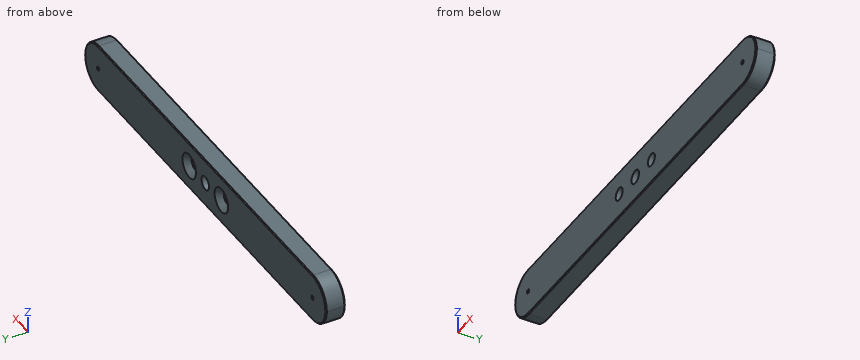
Autodesk Inventor part; units mm, degrees
ref_plane "YZ Plane" through (0, 0, 0) normal (1, 0, 0) x (0, 1, 0)
ref_plane "XZ Plane" through (0, 0, 0) normal (0, 1, 0) x (-1, 0, 0)
ref_plane "XY Plane" through (0, 0, 0) normal (0, 0, 1) x (1, 0, 0)
sketch "Sketch1" plane through (0, 0, 0) normal (0, 1, 0) x (-1, 0, 0)
  line L0 (-112.5, 12.5) -> (112.5, 12.5)
  line L1 (112.5, 12.5) -> (112.5, -12.5)
  line L2 (112.5, -12.5) -> (-112.5, -12.5)
  line L3 (-112.5, -12.5) -> (-112.5, 12.5)
  line L4 (-112.5, 12.5) -> (112.5, -12.5) construction
  line L5 (112.5, 12.5) -> (-112.5, -12.5) construction
  point P0 (0, 0)
  dimension "Length" = 225
  dimension "Width" = 25
extrude "Extrusion1" add sketch "Sketch1" along normal mid plane 10
sketch "Sketch2" plane through (0, 5, 0) normal (0, 1, 0) x (1, 0, 0)
  circle A0 centre (0, 0) radius 3.5
  dimension "d4" = 7
extrude "Extrusion2" cut sketch "Sketch2" against normal up to surface (10 mm away)
sketch "Sketch3" plane through (0, 5, 0) normal (0, 1, 0) x (1, 0, 0)
  circle A0 centre (0, 0) radius 3.5
  point P0 (-15, 0)
  point P1 (15, 0)
  dimension "d7" = 30
  dimension "d8" = 15
hole "Hole1" at (-15, 5, 0) at (15, 5, 0) direction (0, -1, 0) diameter 6.5 end through all countersink diameter 12.6 countersink angle 90
sketch "Sketch4" plane through (0, 5, 0) normal (0, 1, 0) x (1, 0, 0)
  point P0 (0, 0)
  point P1 (-100, 0)
  point P2 (100, 0)
  dimension "d16" = 200
  dimension "d17" = 100
hole "Hole2" at (-100, 5, 0) at (100, 5, 0) direction (0, -1, 0) diameter 2.1211 end through all
fillet "Fillet1" radius 12.5 4 edges at (112.5, 0, 12.5) (112.5, 0, -12.5) (-112.5, 0, 12.5) (-112.5, 0, -12.5)
chamfer "Chamfer1" distance 0.5 angle 45 8 edges at (0, 5, 12.5) (108.839, 5, 8.839) (0, 5, -12.5) (-108.839, 5, 8.839) (0, -5, 12.5) (-108.839, -5, 8.839) (0, -5, -12.5) (108.839, -5, 8.839)
properties part number "Brass Plate" material "Brass, Soft Yellow"
Work out the finished part from the listing and answer in its coordinate system (mm). Give positions to 0.01 mm unless a question says otherwise; leave off trailing zeros. Write each loop counter-clockwise with the first axis right and the second up, starting at its lowest first coordinate (ties: lowest second). Pieces come first, ordered by that corner, then holes. Notation, with made-up numbers: (54.25, 66) -> (81.25, 66) arc R22 ccw to (81.25, 102) -> close; hole circle Ø9 at (-11.75, -26.5). An arc over 180 degrees is marked (long way). Write each question's results on one line, items separated by ' | '.
1. Find section A-A on x = -15. Determine the outline of the cut face in (y, z), and give its area (3 significant figures).
Data:
outline: (-5, -12) -> (-4.5, -12.5) -> (4.5, -12.5) -> (5, -12) -> (5, -6.3) -> (1.95, -3.25) -> (-5, -3.25) -> close; (-5, 3.25) -> (1.95, 3.25) -> (5, 6.3) -> (5, 12) -> (4.5, 12.5) -> (-4.5, 12.5) -> (-5, 12) -> close | area: 175 mm^2
2. Straight lines are drawn through the part: L1, parallel to X at y = -1.75, z = 0; L2, parallel to Z at x = 100, y = 1.5; L3, parallel to X at y = 0.25, z = -0.5. For each, find the intervals that lie inside material, in ascending order.
Data:
L1: -112.5 to -101.06, -98.94 to -18.25, -11.75 to -3.5, 3.5 to 11.75, 18.25 to 98.94, 101.06 to 112.5 | L2: -12.5 to -1.06, 1.06 to 12.5 | L3: -112.49 to -100.94, -99.06 to -18.21, -11.79 to -3.46, 3.46 to 11.79, 18.21 to 99.06, 100.94 to 112.49
3. Each of these flat-tipped pins is pushed along its axis until it touches: pin 1 Ø8 at (x, z) = (17, -1) entering from +Y; pin 2 Ø2 at (y, z) = (-1.5, -7.5) entering from +X; pin 3 Ø1.5 at (y, z) = (-3, 7) entering from -X. Where does it stop, or does it pass through?
Data:
pin 1: y = 4.94 | pin 2: x = 110.68 | pin 3: x = -110.83
4. Find section B-B on y = -0.75. Give the number of separate pieces and of enclosed holes in the cut face, and give its area (3 significant figures).
Data:
separate pieces: 1 | enclosed holes: 5 | area: 5,380 mm^2
